Geometry check sheet. Reference: the model listing, model coordinates, mm. Face numbers are marked on the shaded views. A direction names the side the tool comes from. Round coordinates to 2 decimals unless told otherwise and drop trailing zeros. Write each loop counter-clockwise with the first axis right and the second up, starting at its lowest first coordinate (ties: lowest second). Pieces come first, ordered by that corner, then holes. Notation, with made-up numbers: (63, 59) -> (107, 59) arc R21 ccw to (107, 93) -> close; hole circle Ø8 at (84, 59). An arc over 180 degrees is marked (long way). Use a Markdown table: item, result.
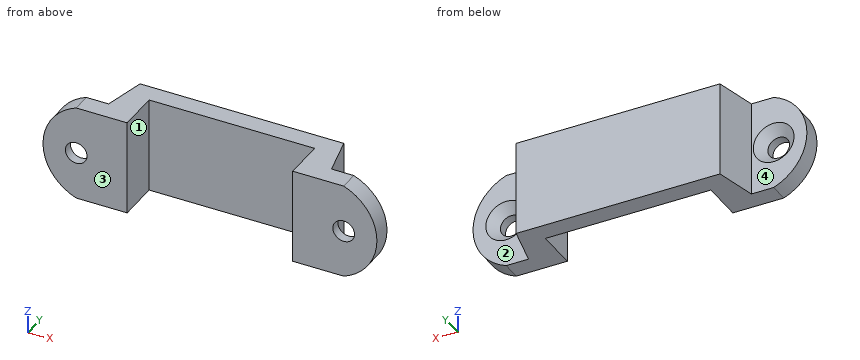
```python
from build123d import *

# Parameters (mm, degrees)
BOSS_EXTRUDE1_DEPTH                                 = 15
BOSS_EXTRUDE2_DEPTH                                 = 3
CSK_FOR_M3_COUNTERSUNK_FLAT_HEAD_SCREW1_D           = 3.4
CSK_FOR_M3_COUNTERSUNK_FLAT_HEAD_SCREW1_DEPTH       = 64
CSK_FOR_M3_COUNTERSUNK_FLAT_HEAD_SCREW1_CSINK_D     = 6.4
CSK_FOR_M3_COUNTERSUNK_FLAT_HEAD_SCREW1_CSINK_ANGLE = 90
CSK_FOR_M3_COUNTERSUNK_FLAT_HEAD_SCREW1_TIP         = 1.021463052


with BuildPart() as part:
    # Sketch2 → Boss-Extrude1 (new body)
    with BuildSketch(Plane.XY):
        Polygon((1.5, 6.5), (0, 0), (-3.5, 0), (-3.5, -3), (4.5, -3), (4.5, 3.5), (30.5, 3.5), (30.5, -3), (38.5, -3), (38.5, 0), (35, 0), (33.5, 6.5), align=None)
    extrude(amount=BOSS_EXTRUDE1_DEPTH)

    # Sketch3 → Boss-Extrude2 (add)
    with BuildSketch(Plane(origin=(0, 0, 0), x_dir=(1, 0, 0), z_dir=(0, 1, 0))):
        with BuildLine():
            Line((-3.5, 0), (-3.5, -15))
            ThreePointArc((-3.5, -15), (-8.716117819, -7.5), (-3.5, 0))
        make_face()
        with BuildLine():
            Line((38.5, 0), (38.5, -15))
            ThreePointArc((38.5, -15), (43.716117819, -7.5), (38.5, 0))
        make_face()
    extrude(amount=-BOSS_EXTRUDE2_DEPTH)

    # CSK for M3 Countersunk Flat Head Screw1
    with Locations(Plane(origin=(0, 0, 0), x_dir=(1, 0, 0), z_dir=(0, 1, 0))):
        with Locations((-3.5, -7.5), (38.5, -7.5)):
            CounterSinkHole(CSK_FOR_M3_COUNTERSUNK_FLAT_HEAD_SCREW1_D / 2, CSK_FOR_M3_COUNTERSUNK_FLAT_HEAD_SCREW1_CSINK_D / 2, depth=CSK_FOR_M3_COUNTERSUNK_FLAT_HEAD_SCREW1_DEPTH, counter_sink_angle=CSK_FOR_M3_COUNTERSUNK_FLAT_HEAD_SCREW1_CSINK_ANGLE)
            with Locations((0, 0, -(CSK_FOR_M3_COUNTERSUNK_FLAT_HEAD_SCREW1_DEPTH + CSK_FOR_M3_COUNTERSUNK_FLAT_HEAD_SCREW1_TIP / 2))):  # 118° drill point
                Cone(0, CSK_FOR_M3_COUNTERSUNK_FLAT_HEAD_SCREW1_D / 2, CSK_FOR_M3_COUNTERSUNK_FLAT_HEAD_SCREW1_TIP, mode=Mode.SUBTRACT)


solid = part.part
```
(1) Section check B-B on y = 1. Record the cut outline in (x, z), plus the area to 3 significant figures.
A:
| item | result |
|---|---|
| outline | (0.23, 0) -> (4.5, 0) -> (4.5, 15) -> (0.23, 15) -> close; (30.5, 0) -> (34.77, 0) -> (34.77, 15) -> (30.5, 15) -> close |
| area | 128 mm2 |
(2) Gauge pin test, flat ends, axial feed: pin 1 Ø3 at (y, z) = (3.5, 11.5) entering from -X; pin 2 Ø4.5 at (x, z) = (-2.5, 7) entering from +Y; pin 3 Ø2 at (y, z) = (1.5, 9.5) entering from +X. Record the tip position at first contact, or that the pin passes through.
A:
| item | result |
|---|---|
| pin 1 | stops at x = 0.46 |
| pin 2 | stops at y = 0 |
| pin 3 | stops at x = 34.88 |
(3) Section check C-C on z = 1.5. Record the cut outline in (x, y).
A:
| item | result |
|---|---|
| outline | (-6.01, -3) -> (4.5, -3) -> (4.5, 3.5) -> (30.5, 3.5) -> (30.5, -3) -> (41.01, -3) -> (41.01, 0) -> (35, 0) -> (33.5, 6.5) -> (1.5, 6.5) -> (0, 0) -> (-6.01, 0) -> close |
(4) Section check D-D on x = 26.5. Record the cut outline in (y, z).
A:
| item | result |
|---|---|
| outline | (3.5, 0) -> (6.5, 0) -> (6.5, 15) -> (3.5, 15) -> close |
(5) Access from +Z, -Z, +X, -X, +Y, -Y to the whole of each face (thin tool, end or side, straight path). Record for the marked faces 1, 2, 3 and 4.
A:
| item | result |
|---|---|
| face 1 | +Z, -Z, -Y |
| face 2 | +Z, -Z, +X, +Y |
| face 3 | +Z, -Z, +X, -X, -Y |
| face 4 | +Z, -Z, -X, +Y |
(6) Section check A-A on z = 7.5. Record the cut outline in (x, y), plus the area to 3 significant figures.
A:
| item | result |
|---|---|
| outline | (-8.72, -3) -> (-5.2, -3) -> (-5.2, -1.5) -> (-6.7, 0) -> (-8.72, 0) -> close; (-1.8, -3) -> (4.5, -3) -> (4.5, 3.5) -> (30.5, 3.5) -> (30.5, -3) -> (36.8, -3) -> (36.8, -1.5) -> (35.3, 0) -> (35, 0) -> (33.5, 6.5) -> (1.5, 6.5) -> (0, 0) -> (-0.3, 0) -> (-1.8, -1.5) -> close; (40.2, -3) -> (43.72, -3) -> (43.72, 0) -> (41.7, 0) -> (40.2, -1.5) -> close |
| area | 181 mm2 |
(7) Thickness scan on line 1 (Z direction, x = -3.5, y = -1.75); line 2 (Y direction, x = 28, z = 7.25); line 3 (X direction, y = 0.5, z = 12.25). Record the ranges inside material, lowest first.
A:
| item | result |
|---|---|
| line 1 | z = 0 to 5.8, 9.2 to 15 |
| line 2 | y = 3.5 to 6.5 |
| line 3 | x = 0.12 to 4.5, 30.5 to 34.88 |
